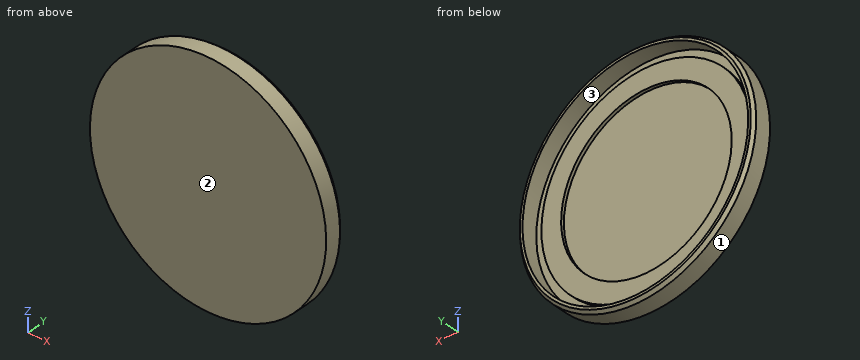
```python
from build123d import *


with BuildPart() as part:
    # Sketch1 → Removable Drainage Saucer (revolve)
    with BuildSketch(Plane.XY, mode=Mode.PRIVATE) as removable_drainage_saucer_sk:
        Polygon((0, 0), (180, 0), (180, 25), (176, 30), (172, 30), (172, 5), (160, 5), (160, 10), (130, 10), (130, 5), (0, 5), align=None)
    revolve(removable_drainage_saucer_sk.sketch.rotate(Axis((0, -10, 0), (0, 1, 0)), 90), axis=Axis((0, -10, 0), (0, 1, 0)))


solid = part.part
```
Geometry check sheet. Reference: the model listing, model coordinates, mm. Face numbers are marked on the shaded views. Round coordinates to 2 decimals unless told otherwise and drop trailing zeros. Order: outer loops, then holes, each group sorted by start corner. A loop starts at its lowest first (then second) coordinate and runs counter-clockwise, first axis right, second up. Notation, with made-up numbers: M 21,-15 L 54,-15 A21 ccw 54,24 Z; hole C -9.75,-18.75 d9. An arc over 180 degrees is marked long. Write item = value, one per line.
Q1. Section check A-A (x = 0). Enter the section's corners in (y, z), plus the area to 3 significant figures.
Answer block:
outline = M 0,-180 L 25,-180 L 30,-176 L 30,-172 L 5,-172 L 5,-160 L 10,-160 L 10,-130 L 5,-130 L 5,130 L 10,130 L 10,160 L 5,160 L 5,172 L 30,172 L 30,176 L 25,180 L 0,180 Z
area = 2,480 mm^2
Q2. Depth check by flat-ended pin: pin 1 Ø10 at (y, z) = (3.5, 14) entering from -X; pin 2 Ø4 at (x, z) = (-87, 132.5) entering from +Y; pin 3 Ø1 at (x, z) = (89.5, -18.5) entering from +Y. Enter the tip coordinate at first touch or a pass-through.
Answer block:
pin_1 = -179.77
pin_2 = 10
pin_3 = 5
Q3. Release check for a two-part mould opening along X. For the marked faces 1, 2 and 3 record: released by +X, released by -X, zero draft, split by the parting line, or undercut.
Answer block:
face_1 = split by the parting line
face_2 = zero draft
face_3 = undercut
Q4. Section check B-B (z = 0). Enter the section's corners in (x, y), plus the area to 3 significant figures.
Answer block:
outline = M -180,0 L 180,0 L 180,25 L 176,30 L 172,30 L 172,5 L 160,5 L 160,10 L 130,10 L 130,5 L -130,5 L -130,10 L -160,10 L -160,5 L -172,5 L -172,30 L -176,30 L -180,25 Z
area = 2,480 mm^2
Q5. Section check C-C (y = 17). Enter the section's corners in (x, z).
Answer block:
outline = C 0,0 d360; hole C 0,0 d344
Q6. Scan lines: line 1 (X direction, y = 6.35, z = 0); line 2 (X direction, y = 9.75, z = -115); line 3 (X direction, y = 25, z = 0). Record each from-to range of solid material in increasing order.
Answer block:
line_1 = -180 to -172, -160 to -130, 130 to 160, 172 to 180
line_2 = -138.47 to -127.9, -111.24 to -60.62, 60.62 to 111.24, 127.9 to 138.47
line_3 = -180 to -172, 172 to 180
